The model under review builds one solid part; all positions refer to its coordinate system, in mm. Face numbers are marked on the shaded views. A direction names the side the tool comes from. Coordinates: 2 decimals unless noted, no trailing zeros. Order: outer loops, then holes, each group sorted by start corner. A loop starts at its lowest first (then second) coordinate and runs counter-clockwise, first axis right, second up. Notation, with made-up numbers: (69, 34.5) -> (94, 34.5) arc R14 cw to (94, 46.5) -> close; hole circle Ø5 at (-17, -6.5). An arc over 180 degrees is marked (long way). Put each result on its own line as item: value.
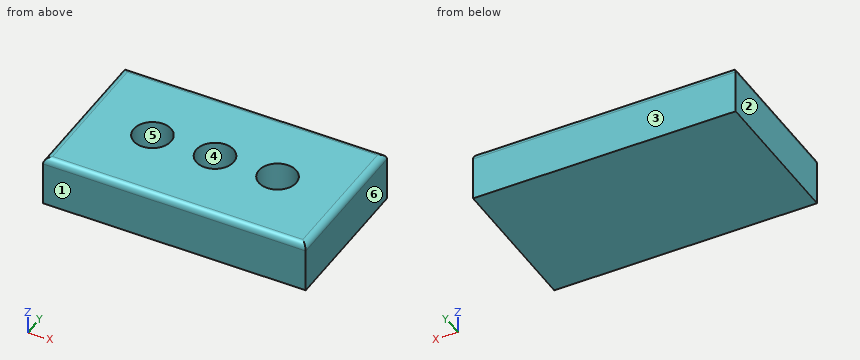
from build123d import *

# Parameters (mm, degrees)
F0_W     = 105
F0_H     = 60
F1_DEPTH = 20
F2_R     = 7.5
F3_DEPTH = 15
F4_R     = 2.5


with BuildPart() as f1:
    # F0 (on Top) → F1 (new body)
    with BuildSketch(Plane.XY):
        Rectangle(F0_W, F0_H)
    extrude(amount=F1_DEPTH)

    # F2 (on face) → F3 (cut)
    with BuildSketch(Plane.XY.offset(20)):
        with Locations((-25, 0)):
            Circle(F2_R)
        with Locations((25, 0)):
            Circle(F2_R)
        Circle(F2_R)
    extrude(amount=-F3_DEPTH, mode=Mode.SUBTRACT)

    # F4
    f4_edges = [f1.edges().sort_by_distance(p)[0] for p in [
        (-52.5, 0, 20),
        (0, 30, 20),
        (52.5, 0, 20),
        (0, -30, 20),
    ]]
    fillet(f4_edges, radius=F4_R)


solid = f1.part
Item 1: Consider section B-B on y = 0. Write out the cut boundary in (x, z).
Answers below:
outline: (-52.5, 0) -> (52.5, 0) -> (52.5, 17.5) arc R2.5 ccw to (50, 20) -> (32.5, 20) -> (32.5, 5) -> (17.5, 5) -> (17.5, 20) -> (7.5, 20) -> (7.5, 5) -> (-7.5, 5) -> (-7.5, 20) -> (-17.5, 20) -> (-17.5, 5) -> (-32.5, 5) -> (-32.5, 20) -> (-50, 20) arc R2.5 ccw to (-52.5, 17.5) -> close
Item 2: For the marked faces 5 and 6, list the 3-axis set-ups (+Z, -Z, +X, -X, +Y, -Y) from which the entire face can be reached by the end or side of a thin tool; tool diameter is ignored.
Answers below:
face 5: +Z
face 6: +Z, -Z, +X, +Y, -Y
Item 3: Consider section D-D on x = 28.5. Write out the cut boundary in (y, z).
Answers below:
outline: (-30, 0) -> (30, 0) -> (30, 17.5) arc R2.5 ccw to (27.5, 20) -> (6.63, 20) -> (6.63, 5) -> (-6.63, 5) -> (-6.63, 20) -> (-27.5, 20) arc R2.5 ccw to (-30, 17.5) -> close
Item 4: Mouldability with a two-part tool opening along Y and no side actions: class the marked faces 1, 2, 3 and 4 as +Y half, -Y half, draft (parallel to the pull), parting line (faces both ways), or undercut.
Answers below:
face 1: -Y half
face 2: draft
face 3: +Y half
face 4: undercut
Item 5: Consider section C-C on x = -25. Write out the cut boundary in (y, z).
Answers below:
outline: (-30, 0) -> (30, 0) -> (30, 17.5) arc R2.5 ccw to (27.5, 20) -> (7.5, 20) -> (7.5, 5) -> (-7.5, 5) -> (-7.5, 20) -> (-27.5, 20) arc R2.5 ccw to (-30, 17.5) -> close
Item 6: Consider section A-A on z = 9.75. Write out the cut boundary in (x, y).
Answers below:
outline: (-52.5, -30) -> (52.5, -30) -> (52.5, 30) -> (-52.5, 30) -> close; hole circle Ø15 at (-25, 0); hole circle Ø15 at (0, 0); hole circle Ø15 at (25, 0)
Item 7: For pin 1 Ø10 at (x, y) = (-13, -14) entering from -Z; pin 2 Ø2 at (x, y) = (22, -4.5) entering from +Z, all flat-tipped, find the tip position at first contact; note any pin that passes through.
Answers below:
pin 1: z = 0
pin 2: z = 5
Item 8: For line 1 (X direction, y = 6, z = 7); line 2 (Z direction, x = -5, y = 4.5); line 3 (Y direction, x = 0, z = 9.5), list the stretches that pass through material, from the lowest coordinate up. Write a range as from..to.
Answers below:
line 1: -52.5..-29.5, -20.5..-4.5, 4.5..20.5, 29.5..52.5
line 2: 0..5
line 3: -30..-7.5, 7.5..30
